Read the model definition and answer for the solid it produces. Units are mm, in the model's axes. Face numbers are marked on the shaded views. A direction names the side the tool comes from. Give positions to 0.01 mm unless a question says otherwise; leave off trailing zeros. Write each loop counter-clockwise with the first axis right and the second up, starting at its lowest first coordinate (ties: lowest second). Pieces come first, ordered by that corner, then holes. Notation, with made-up numbers: (4.25, 17.5) -> (36.25, 17.5) arc R19 ccw to (36.25, 33.5) -> close; hole circle Ø2 at (70, -33). An arc over 180 degrees is marked (long way). Write item = value, one per line.
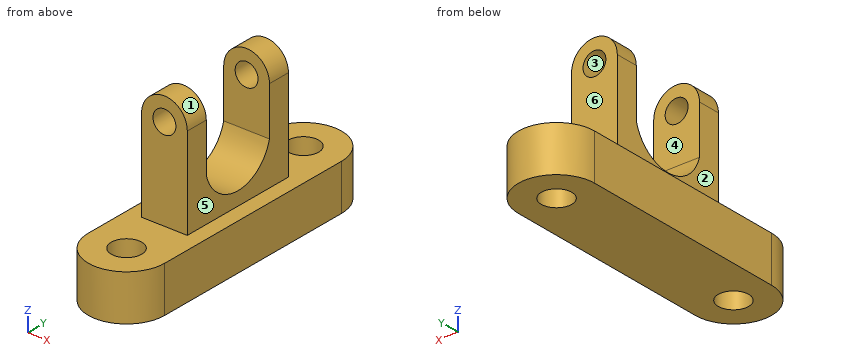
from build123d import *

# Parameters (mm, degrees)
F1_DEPTH = 19.05
F2_R     = 6.35
F3_DEPTH = 25.4
F5_DEPTH = 25.4
F6_R     = 4.7625
F7_DEPTH = 50.8
F9_DEPTH = 25.4


with BuildPart() as f1:
    # F0 (on Top) → F1 (new body)
    with BuildSketch(Plane.XY):
        with BuildLine():
            ThreePointArc((-15.875, 44.45), (0, 28.575), (15.875, 44.45))
            Line((15.875, 44.45), (-15.875, 44.45))
        make_face()
        with BuildLine():
            Line((-15.875, 44.45), (15.875, 44.45))
            ThreePointArc((15.875, 44.45), (0, 60.325), (-15.875, 44.45))
        make_face()
        with BuildLine():
            Line((15.875, -44.45), (15.875, 44.45))
            ThreePointArc((15.875, 44.45), (0, 28.575), (-15.875, 44.45))
            Line((-15.875, 44.45), (-15.875, -44.45))
            ThreePointArc((-15.875, -44.45), (0, -28.575), (15.875, -44.45))
        make_face()
        with BuildLine():
            ThreePointArc((-15.875, -44.45), (0, -60.325), (15.875, -44.45))
            Line((15.875, -44.45), (-15.875, -44.45))
        make_face()
        with BuildLine():
            Line((-15.875, -44.45), (15.875, -44.45))
            ThreePointArc((15.875, -44.45), (0, -28.575), (-15.875, -44.45))
        make_face()
    extrude(amount=F1_DEPTH)

    # F2 (on face) → F3 (cut)
    with BuildSketch(Plane.XY.offset(19.05)):
        with Locations((0, -44.45)):
            Circle(F2_R)
        with Locations((0, 44.45)):
            Circle(F2_R)
    extrude(amount=-F3_DEPTH, mode=Mode.SUBTRACT)

    # F4 (on Front) → F5 (join, symmetric)
    with BuildSketch(Plane.XZ):
        with BuildLine():
            Line((-9.525, 57.15), (-9.525, 19.05))
            Line((-9.525, 19.05), (9.525, 19.05))
            Line((9.525, 19.05), (9.525, 57.15))
            ThreePointArc((9.525, 57.15), (0, 47.625), (-9.525, 57.15))
        make_face()
        with BuildLine():
            ThreePointArc((9.525, 57.15), (0, 66.675), (-9.525, 57.15))
            Line((-9.525, 57.15), (9.525, 57.15))
        make_face()
        with BuildLine():
            Line((9.525, 57.15), (-9.525, 57.15))
            ThreePointArc((-9.525, 57.15), (0, 47.625), (9.525, 57.15))
        make_face()
    extrude(amount=F5_DEPTH, both=True)

    # F6 (on face) → F7 (cut, through all)
    with BuildSketch(Plane.XZ.offset(25.4)):
        with Locations((0, 57.15)):
            Circle(F6_R)
    extrude(amount=-F7_DEPTH, mode=Mode.SUBTRACT)

    # F8 (on face) → F9 (cut)
    with BuildSketch(Plane.YZ.offset(9.525)):
        with BuildLine():
            Line((15.875, 71.8479231), (0, 71.8479231))
            Line((0, 71.8479231), (-15.875, 71.8479231))
            Line((-15.875, 71.8479231), (-15.875, 45.2380125161))
            ThreePointArc((-15.875, 45.2380125161), (0, 57.496732945), (15.875, 45.2380125161))
            Line((15.875, 45.2380125161), (15.875, 71.8479231))
        make_face()
        with BuildLine():
            ThreePointArc((15.875, 45.2380125161), (0, 57.496732945), (-15.875, 45.2380125161))
            Line((-15.875, 45.2380125161), (-15.875, 36.9386635721))
            Line((-15.875, 36.9386635721), (15.875, 36.9386635721))
            Line((15.875, 36.9386635721), (15.875, 45.2380125161))
        make_face()
        with BuildLine():
            Line((15.875, 36.9386635721), (-15.875, 36.9386635721))
            ThreePointArc((-15.875, 36.9386635721), (0, 24.6799431432), (15.875, 36.9386635721))
        make_face()
    extrude(amount=-F9_DEPTH, mode=Mode.SUBTRACT)


solid = f1.part
(1) Consider L1, parallel to Z at x = 0, y = 22.25 (1 decimal); L2, parallel to Y at x = 9, z = 50 (3 decimals); L3, parallel to Z at x = 2.5, y = -27.5. Determine where each line is inside the solid, lowest interval first.
Checks:
L1 = 0 to 52.4, 61.9 to 66.7
L2 = -25.4 to -15.875, 15.875 to 25.4
L3 = 0 to 19.05
(2) A tool of negligible diameter and unlimited length cuts with its end or side. For the marked faces 4, 5 and 6, from which of +Z, -Z, +X, -X, +Y, -Y can it reach the whole face along a straight path? Write none if from no direction.
Checks:
face_4 = +Z, +X, -X
face_5 = +Z, +X, +Y, -Y
face_6 = +Z, +X, -X, +Y
(3) The part is cut by section D-D on y = 42.5. Determine the outline of the cut face in (x, z) (3 decimals).
Checks:
outline = (-15.875, 0) -> (-6.043, 0) -> (-6.043, 19.05) -> (-15.875, 19.05) -> close; (6.043, 0) -> (15.875, 0) -> (15.875, 19.05) -> (6.043, 19.05) -> close
(4) The part is cut by section C-C on z = 59.5. Determine the outline of the cut face in (x, y) (3 decimals), plus the area to 3 significant figures.
Checks:
outline = (-9.231, -25.4) -> (-4.142, -25.4) -> (-4.142, -15.875) -> (-9.231, -15.875) -> close; (-9.231, 15.875) -> (-4.142, 15.875) -> (-4.142, 25.4) -> (-9.231, 25.4) -> close; (4.142, -25.4) -> (9.231, -25.4) -> (9.231, -15.875) -> (4.142, -15.875) -> close; (4.142, 15.875) -> (9.231, 15.875) -> (9.231, 25.4) -> (4.142, 25.4) -> close
area = 194 mm²
(5) The part is cut by section A-A on x = 0. Count the separate pieces of the cut face and the enclosed holes in it, plus the area to 3 significant figures.
Checks:
separate_pieces = 5
enclosed_holes = 0
area = 2,820 mm²
(6) For a pull along Z with two mould halves and no side action, classify the marked faces 1, 2 and 3 as released by +Z, released by -Z, zero draft, split by the parting line, or undercut.
Checks:
face_1 = released by +Z
face_2 = zero draft
face_3 = undercut
(7) Given P1, Ø5.5, axis at x = 0.5, z = 52, coming from the +Y side; P2, Ø5, axis at x = -9, z = 44.5, coming from the -Y side; P3, Ø3, axis at x = 1, y = -3.5, coming from the +Z side, each flat-ended and moving along its own axis, determine where each tip first touches the part or whether it passes through.
Checks:
P1 = 25.4
P2 = -25.4
P3 = 25.46
